Here's how the part is built. I have some questions about the finished solid (model axes, mm). A direction names the side the tool comes from. Coordinates: 2 decimals unless noted, no trailing zeros. Write each loop counter-clockwise with the first axis right and the second up, starting at its lowest first coordinate (ties: lowest second). Pieces come first, ordered by that corner, then holes. Notation, with made-up numbers: M -19,69.5 L -11,69.5 A23 ccw -11,90.5 Z; hole C -28,-25.5 d1. An arc over 180 degrees is marked long. Use a Markdown table: item, result.
```python
from build123d import *

# Parameters (mm, degrees)
ESQUISSE1_W             = 26
ESQUISSE1_H             = 28
BOSS_EXTRU_1_DEPTH      = 8
ENL_V_MAT_EXTRU_1_DEPTH = 9
ENL_V_MAT_EXTRU_2_DEPTH = 4.2
ESQUISSE4_R             = 1.7
ENL_V_MAT_EXTRU_3_DEPTH = 9
ESQUISSE5_R             = 3.3
ENL_V_MAT_EXTRU_6_DEPTH = 4.2
ESQUISSE6_R             = 1.7
BOSS_EXTRU_2_DEPTH      = 1
ESQUISSE7_R             = 3
ESQUISSE7_R_2           = 1.7
BOSS_EXTRU_3_DEPTH      = 1.5
FILLET1_R               = 2


with BuildPart() as part:
    # Esquisse1 → Boss.-Extru.1 (new body)
    with BuildSketch(Plane.XY):
        with Locations((5, 0)):
            Rectangle(ESQUISSE1_W, ESQUISSE1_H)
    extrude(amount=BOSS_EXTRU_1_DEPTH)

    # Esquisse2 → Enlèv. mat.-Extru.1 (cut, through all)
    with BuildSketch(Plane.XY.offset(8)):
        with BuildLine():
            Line((-0.8, 8), (-0.8, -8))
            ThreePointArc((-0.8, -8), (-3, -10.2), (-5.2, -8))
            Line((-5.2, -8), (-5.2, 8))
            ThreePointArc((-5.2, 8), (-3, 10.2), (-0.8, 8))
        make_face()
    extrude(amount=-ENL_V_MAT_EXTRU_1_DEPTH, mode=Mode.SUBTRACT)

    # Esquisse3 → Enlèv. mat.-Extru.2 (cut)
    with BuildSketch(Plane.XY.offset(8)):
        with BuildLine():
            Line((1, 8), (1, -8))
            ThreePointArc((1, -8), (-3, -12), (-7, -8))
            Line((-7, -8), (-7, 8))
            ThreePointArc((-7, 8), (-3, 12), (1, 8))
        make_face()
    extrude(amount=-ENL_V_MAT_EXTRU_2_DEPTH, mode=Mode.SUBTRACT)

    # Esquisse4 → Enlèv. mat.-Extru.3 (cut, through all)
    with BuildSketch(Plane.XY.offset(8)):
        with Locations((15, 9.25)):
            Circle(ESQUISSE4_R)
        with Locations((15, -9.25)):
            Circle(ESQUISSE4_R)
    extrude(amount=-ENL_V_MAT_EXTRU_3_DEPTH, mode=Mode.SUBTRACT)

    # Esquisse5 → Enlèv. mat.-Extru.6 (cut)
    with BuildSketch(Plane(origin=(0, 0, 0), x_dir=(-1, 0, 0), z_dir=(0, 0, -1))):
        with Locations((-15, 9.25)):
            Circle(ESQUISSE5_R)
        with Locations((-15, -9.25)):
            Circle(ESQUISSE5_R)
    extrude(amount=-ENL_V_MAT_EXTRU_6_DEPTH, mode=Mode.SUBTRACT)

    # Esquisse6 → Boss.-Extru.2 (add)
    with BuildSketch(Plane(origin=(0, 0, 4.2), x_dir=(-1, 0, 0), z_dir=(0, 0, -1))):
        with Locations((-15, 9.25)):
            Circle(ESQUISSE6_R)
        with Locations((-15, -9.25)):
            Circle(ESQUISSE6_R)
    extrude(amount=-BOSS_EXTRU_2_DEPTH)

    # Esquisse7 → Boss.-Extru.3 (add)
    with BuildSketch(Plane.XY.offset(8)):
        with Locations((15, -9.25)):
            Circle(ESQUISSE7_R)
        with Locations((15, -9.25)):
            Circle(ESQUISSE7_R_2, mode=Mode.SUBTRACT)
        with Locations((15, 9.25)):
            Circle(ESQUISSE7_R)
        with Locations((15, 9.25)):
            Circle(ESQUISSE7_R_2, mode=Mode.SUBTRACT)
    extrude(amount=BOSS_EXTRU_3_DEPTH)

    # Fillet1
    fillet1_edges = [part.edges().sort_by_distance(p)[0] for p in [
        (-8, 14, 4),
        (18, 14, 4),
        (18, -14, 4),
        (-8, -14, 4),
    ]]
    fillet(fillet1_edges, radius=FILLET1_R)


solid = part.part
```
1. Suppose I cut it at D-D on y = -11.5. Write out the boundary of the cut face in (x, z), and give its area (3 significant figures).
Answers follow:
| item | result |
|---|---|
| outline | M -8,0 L 12.59,0 L 12.59,4.2 L 17.41,4.2 L 17.41,0 L 18,0 L 18,8 L 16.98,8 L 16.98,9.5 L 13.02,9.5 L 13.02,8 L -1.06,8 L -1.06,3.8 L -4.94,3.8 L -4.94,8 L -8,8 Z |
| area | 177 mm2 |
2. We'd pull the mould along Y, two halves only. Please class faces 1 (the face through (-7.4, -13.43, 4.06)), 2 (the face through (16.57, -9.9, 7.32)), 3 (the face through (-8, 0, 4)): +Y half, -Y half, draft (parallel to the pull), parting line (faces both ways), or undercut.
Answers follow:
| item | result |
|---|---|
| face 1 | -Y half |
| face 2 | undercut |
| face 3 | draft |
3. Will these pins go through, and if not, where does the flat tip stop? pin 1 Ø6 at (x, y) = (4, -5) entering from +Z; pin 2 Ø2.5 at (x, y) = (15, -9.5) entering from +Z; pin 3 Ø1.5 at (x, y) = (-5, -9) entering from +Z; pin 4 Ø2 at (x, y) = (-2, 7.5) entering from +Z.
Answers follow:
| item | result |
|---|---|
| pin 1 | stops at z = 8 |
| pin 2 | stops at z = 5.2 |
| pin 3 | stops at z = 3.8 |
| pin 4 | passes through |
4. Which directions (+Z, -Z, +X, -X, +Y, -Y) give clear straight access to the entire face, cutting with the end or side of a thin tool? Please do faces 4 (the face through (15, -9, 4.2)), 5 (the face through (5, -14, 4)), 6 (the face through (18, 0, 4)), 7 (the face through (12.79, -7.22, 8.74)), 8 (the face through (-5.2, 0, 2)).
Answers follow:
| item | result |
|---|---|
| face 4 | -Z |
| face 5 | +Z, -Z, +X, -X, -Y |
| face 6 | +Z, -Z, +X, +Y, -Y |
| face 7 | +Z |
| face 8 | +Z, -Z |
5. Suppose I cut it at B-B on x = -3. Write out the boundary of the cut face in (y, z), and give its area (3 significant figures).
Answers follow:
| item | result |
|---|---|
| outline | M -14,0 L -10.2,0 L -10.2,3.8 L -12,3.8 L -12,8 L -14,8 Z; M 10.2,0 L 14,0 L 14,8 L 12,8 L 12,3.8 L 10.2,3.8 Z |
| area | 45.7 mm2 |
6. I need wall thicknesses on probe 1 along Y at (x, z) = (15, 6.8); probe 2 along Y at (x, z) = (15, 0.95); probe 3 along X at (y, z) = (-9.25, 7.8). Which ranges of each line are inside material? Lowest first, please.
Answers follow:
| item | result |
|---|---|
| probe 1 | y = -14 to -10.95, -7.55 to 7.55, 10.95 to 14 |
| probe 2 | y = -14 to -12.55, -5.95 to 5.95, 12.55 to 14 |
| probe 3 | x = -8 to -6.8, 0.8 to 13.3, 16.7 to 18 |
7. Suppose I cut it at A-A on z = 7. Write out the boundary of the cut face in (x, y).
Answers follow:
| item | result |
|---|---|
| outline | M -8,-12 A2 ccw -6,-14 L 16,-14 A2 ccw 18,-12 L 18,12 A2 ccw 16,14 L -6,14 A2 ccw -8,12 Z; hole M -7,-8 A4 ccw 1,-8 L 1,8 A4 ccw -7,8 Z; hole C 15,-9.25 d3.4; hole C 15,9.25 d3.4 |
8. Suppose I cut it at C-C on z = 2. Write out the boundary of the cut face in (x, y), and give its area (3 significant figures).
Answers follow:
| item | result |
|---|---|
| outline | M -8,-12 A2 ccw -6,-14 L 16,-14 A2 ccw 18,-12 L 18,-10.62 A3.3 cw long 18,-7.88 L 18,7.88 A3.3 cw long 18,10.62 L 18,12 A2 ccw 16,14 L -6,14 A2 ccw -8,12 Z; hole M -5.2,-8 A2.2 ccw -0.8,-8 L -0.8,8 A2.2 ccw -5.2,8 Z |
| area | 572 mm2 |
